```python
from build123d import *

# Parameters (mm, degrees)
SKETCH1_R                                = 7
DA_CIRCLE_DEPTH                          = 2.5
ONE_TEETH_DEPTH                          = 11.210288928
FILLET_FOR_HIGH_R                        = 0.5
CIRPATTERN_FOR_HIGH_COUNT                = 12
FILLET_FOR_HIGH_OF_CIRPATTERN_FOR_HIGH_R = 0.5


with BuildPart() as part:
    # Sketch1 → Da_circle (new, symmetric)
    with BuildSketch(Plane.XY):
        Circle(SKETCH1_R)
    extrude(amount=DA_CIRCLE_DEPTH, both=True)

    # Sketch → one_teeth (cut, symmetric)
    with BuildSketch(Plane.XY):
        with BuildLine():
            ThreePointArc((-0.54138974, 4.719046212), (0, 4.75), (0.54138974, 4.719046212))
            Line((0.54138974, 4.719046212), (0.642618876, 5.601414192))
            ThreePointArc((0.642618876, 5.601414192), (0.704564548, 5.778410288), (0.783157153, 5.948669168))
            ThreePointArc((0.783157153, 5.948669168), (1.15155426, 6.444705558), (1.656172795, 6.801256625))
            ThreePointArc((1.656172795, 6.801256625), (0, 7), (-1.656172795, 6.801256625))
            ThreePointArc((-1.656172795, 6.801256625), (-1.02382272, 6.30741194), (-0.642618876, 5.601414192))
            Line((-0.642618876, 5.601414192), (-0.54138974, 4.719046212))
        make_face()
    one_teeth = extrude(amount=ONE_TEETH_DEPTH, both=True, mode=Mode.SUBTRACT)

    # Fillet_for_high
    fillet_for_high_edges = [part.edges().sort_by_distance(p)[0] for p in [
        (0.54138974, 4.719046212, 0),
        (-0.54138974, 4.719046212, 0),
    ]]
    fillet(fillet_for_high_edges, radius=FILLET_FOR_HIGH_R)

    # CirPattern_for_high: one_teeth ×12 about axis
    cirpattern_for_high_axis = Axis((0, 0, 0), (0, 0, 1))
    for i in range(1, CIRPATTERN_FOR_HIGH_COUNT):
        add(one_teeth.rotate(cirpattern_for_high_axis, i * 360 / CIRPATTERN_FOR_HIGH_COUNT), mode=Mode.SUBTRACT)

    # Fillet_for_high of CirPattern_for_high
    fillet_for_high_of_cirpattern_for_high_edges = [part.edges().sort_by_distance(p)[0] for p in [
        (-1.890665838, 4.357508771, 0),
        (-2.828380374, 3.816119031, 0),
        (-3.816119031, 2.828380374, 0),
        (-4.357508771, 1.890665838, 0),
        (-4.719046212, 0.54138974, 0),
        (-4.719046212, -0.54138974, 0),
        (-4.357508771, -1.890665838, 0),
        (-3.816119031, -2.828380374, 0),
        (-2.828380374, -3.816119031, 0),
        (-1.890665838, -4.357508771, 0),
        (-0.54138974, -4.719046212, 0),
        (0.54138974, -4.719046212, 0),
        (1.890665838, -4.357508771, 0),
        (2.828380374, -3.816119031, 0),
        (3.816119031, -2.828380374, 0),
        (4.357508771, -1.890665838, 0),
        (4.719046212, -0.54138974, 0),
        (4.719046212, 0.54138974, 0),
        (4.357508771, 1.890665838, 0),
        (3.816119031, 2.828380374, 0),
        (2.828380374, 3.816119031, 0),
        (1.890665838, 4.357508771, 0),
    ]]
    fillet(fillet_for_high_of_cirpattern_for_high_edges, radius=FILLET_FOR_HIGH_OF_CIRPATTERN_FOR_HIGH_R)


solid = part.part
```
Design review of the part built by this model. Coordinates are the model's own, in mm. A direction names the side the tool comes from. Give positions to 0.01 mm unless a question says otherwise; leave off trailing zeros. Order: outer loops, then holes, each group sorted by start corner. A loop starts at its lowest first (then second) coordinate and runs counter-clockwise, first axis right, second up. Notation, with made-up numbers: (63, -1) - (84, -1) arc R38 ccw to (84, 37) - close; hole circle Ø11 at (69.5, 59). An arc over 180 degrees is marked (long way). Use a Markdown table: item, result. Add a question column.
(1) Add section A-A on y = -6. Give the boundary of the cut face in (x, z).
(2) Add section B-B on y = -1.25. Give the boundary of the cut face in (x, z), then the cut area to 3 significant figures.
(3) Clearance check with a flat-ended pin moving along its axis: P1, Ø2, axis at y = -4.5, z = 1.5, coming from the -X side. State where the tip first meets the part, or that it passes through.
(4) Add section C-C on x = -0.25. Give the boundary of the cut face in (y, z), then the cut area to 3 significant figures.
(5) Wall thickness on probe 1 along Y at (x, z) = (-4.25, 1.65); probe 2 along Y at (x, z) = (-4.5, -0.5); probe 3 along X at (y, z) = (5.5, -0.45): over which ranges is each line inside the solid? List them lowest first. Write a range as [from, to].
(6) Mouldability with a two-part tool opening along X and no side actions: class faces 5 (the face through (1.02, 6.3, 0.04)), 6 (the face through (-2.265, -5.985, 0.035)), 7 (the face through (4.954, 4.051, 0.035)) as +X half, -X half, draft (parallel to the pull), parting line (faces both ways), or undercut.
(7) Machinability: for faces 1 (the face through (-4.051, 4.954, 0.035)), 2 (the face through (1.031, -6.316, 0.035)), 3 (the face through (-6.316, -1.031, 0.035)), 4 (the face through (6.3, -1.02, 0.04)), which of the approach directions +Z, -Z, +X, -X, +Y, -Y give a long, thin tool a straight path to every point of the face, cutting with its end or side? Answer none if there is none.
Report:
| question | item | result |
|---|---|---|
| 1 | outline | (-2.26, -2.5) - (-0.81, -2.5) - (-0.81, 2.5) - (-2.26, 2.5) - close; (0.81, -2.5) - (2.26, -2.5) - (2.26, 2.5) - (0.81, 2.5) - close |
| 2 | outline | (-6.53, -2.5) - (6.53, -2.5) - (6.53, 2.5) - (-6.53, 2.5) - close |
| 2 | area | 65.3 mm² |
| 3 | P1 | stops at x = -5.07 |
| 4 | outline | (-4.77, -2.5) - (4.77, -2.5) - (4.77, 2.5) - (-4.77, 2.5) - close |
| 4 | area | 47.7 mm² |
| 5 | probe 1 | y = [-5.01, -3.15], [-2.18, 2.18], [3.15, 5.01] |
| 5 | probe 2 | y = [-5.06, -3.34], [-2.05, 2.05], [3.34, 5.06] |
| 5 | probe 3 | x = [-2.29, -0.63], [0.63, 2.29] |
| 6 | face 5 | undercut |
| 6 | face 6 | -X half |
| 6 | face 7 | +X half |
| 7 | face 1 | +Z, -Z, +Y |
| 7 | face 2 | +Z, -Z, -Y |
| 7 | face 3 | +Z, -Z, -X |
| 7 | face 4 | +Z, -Z, +X |
